Autodesk Inventor part; units mm, degrees
ref_plane "YZ Plane" through (0, 0, 0) normal (1, 0, 0) x (0, 1, 0)
ref_plane "XZ Plane" through (0, 0, 0) normal (0, 1, 0) x (-1, 0, 0)
ref_plane "XY Plane" through (0, 0, 0) normal (0, 0, 1) x (1, 0, 0)
sketch "Sketch12" plane through (0, 0, 0) normal (0, 0, 1) x (1, 0, 0)
  line L0 (-49, -21) -> (49, -21)
  line L1 (-49, 21) -> (-49, 9)
  line L2 (-49, -9) -> (-52, -9)
  line L3 (-52, -9) -> (-52, -3.75)
  line L4 (-52, 9) -> (-49, 9)
  line L5 (-49, -3.75) -> (-52, -3.75)
  line L6 (-49, 3.75) -> (-52, 3.75)
  line L7 (-44, -1.5) -> (-44, 1.5)
  line L8 (-49, 1.5) -> (-49, -1.5)
  line L9 (-49, -3.75) -> (-49, -9)
  line L10 (-49, 1.5) -> (-49, -1.5)
  line L11 (-49, 3.75) -> (-49, 1.5)
  line L12 (-47, -1.5) -> (-47, -2.65)
  line L13 (-44.6, -2.65) -> (-47, -2.65)
  line L14 (-44.6, -2.65) -> (-44.6, -1.5)
  line L15 (-44.6, 1.5) -> (-44.6, 2.65)
  line L16 (-47, 2.65) -> (-44.6, 2.65)
  line L17 (-47, 1.5) -> (-47, 2.65)
  line L18 (-49, -1.5) -> (-47, -1.5)
  line L19 (-44.6, -1.5) -> (-44, -1.5)
  line L20 (-44, 1.5) -> (-44.6, 1.5)
  line L21 (-47, 1.5) -> (-49, 1.5)
  line L22 (0, -30) -> (0, 33) construction
  line L23 (33.1667, 21) -> (33.1667, 24)
  line L24 (33.1667, 24) -> (5, 24)
  line L25 (-33.1667, 24) -> (-33.1667, 21)
  line L26 (-33.1667, 21) -> (-49, 21)
  line L27 (33.1667, 21) -> (49, 21)
  line L28 (-5, 21) -> (-5, 24)
  line L29 (5, 21) -> (5, 24)
  line L30 (-1.5, 21) -> (-1.5, 19)
  line L31 (-2.65, 19) -> (-1.5, 19)
  line L32 (-2.65, 19) -> (-2.65, 16.6)
  line L33 (-2.65, 16.6) -> (-1.5, 16.6)
  line L34 (-1.5, 16.6) -> (-1.5, 16)
  line L35 (-1.5, 16) -> (1.5, 16)
  line L36 (1.5, 16) -> (1.5, 16.6)
  line L37 (2.65, 16.6) -> (1.5, 16.6)
  line L38 (2.65, 16.6) -> (2.65, 19)
  line L39 (1.5, 19) -> (2.65, 19)
  line L40 (1.5, 19) -> (1.5, 21)
  line L41 (1.5, 21) -> (5, 21)
  line L42 (-5, 24) -> (-33.1667, 24)
  line L43 (5, 24) -> (-5, 24)
  line L44 (-1.5, 21) -> (-5, 21)
  circle A0 centre (0, 0) radius 11.5
  circle A1 centre (32, 0) radius 3.9
  circle A2 centre (-32, 0) radius 3.9
  line L45 (2.65, 19) -> (2.65, 16.6)
  line L46 (2.65, 16.6) -> (-2.65, 16.6)
  line L47 (-2.65, 16.6) -> (-2.65, 19)
  line L48 (-2.65, 19) -> (2.65, 19)
  line L49 (44.6, 2.65) -> (47, 2.65)
  line L50 (47, 2.65) -> (47, -2.65)
  line L51 (47, -2.65) -> (44.6, -2.65)
  line L52 (44.6, -2.65) -> (44.6, 2.65)
  line L53 (-44.6, 2.65) -> (-44.6, -2.65)
  line L54 (-44.6, -2.65) -> (-47, -2.65)
  line L55 (-47, -2.65) -> (-47, 2.65)
  line L56 (-47, 2.65) -> (-44.6, 2.65)
  circle A3 centre (-15.5, -15.5) radius 1.4
  circle A4 centre (-15.5, 15.5) radius 1.4
  circle A5 centre (15.5, 15.5) radius 1.4
  circle A6 centre (15.5, -15.5) radius 1.4
  line L57 (-52, -21) -> (52, -21)
  line L58 (52, -21) -> (52, -10.5)
  line L59 (52, -10.5) -> (49, -10.5)
  line L60 (49, -10.5) -> (49, 10.5)
  line L61 (49, 10.5) -> (52, 10.5)
  line L62 (52, 10.5) -> (52, 24)
  line L63 (52, 24) -> (34.6667, 24)
  line L64 (34.6667, 24) -> (34.6667, 21)
  line L65 (34.6667, 21) -> (-34.6667, 21)
  line L66 (-34.6667, 21) -> (-34.6667, 24)
  line L67 (-34.6667, 24) -> (-52, 24)
  line L68 (-52, 24) -> (-52, 10.5)
  line L69 (-52, 10.5) -> (-49, 10.5)
  line L70 (-49, 10.5) -> (-49, -10.5)
  line L71 (-49, -10.5) -> (-52, -10.5)
  line L72 (-52, -10.5) -> (-52, -21)
  line L73 (-52, -3.75) -> (-52, 3.75)
  line L74 (-52, 3.75) -> (-52, 9)
  line L75 (-72.8, 0) -> (72.8, 0) construction
  line L76 (-49, -9) -> (-49, -21)
  line L77 (-49, 9) -> (-49, 3.75)
  line L78 (-49, -1.5) -> (-49, -3.75)
  line L79 (49, 21) -> (49, 9)
  line L80 (49, -9) -> (52, -9)
  line L81 (52, -9) -> (52, -3.75)
  line L82 (52, 9) -> (49, 9)
  line L83 (49, -3.75) -> (52, -3.75)
  line L84 (49, 3.75) -> (52, 3.75)
  line L85 (44, -1.5) -> (44, 1.5)
  line L86 (49, -3.75) -> (49, -9)
  line L87 (49, 1.5) -> (49, -1.5)
  line L88 (49, 3.75) -> (49, 1.5)
  line L89 (47, -1.5) -> (47, -2.65)
  line L90 (44.6, -2.65) -> (47, -2.65)
  line L91 (44.6, -2.65) -> (44.6, -1.5)
  line L92 (44.6, 1.5) -> (44.6, 2.65)
  line L93 (47, 2.65) -> (44.6, 2.65)
  line L94 (47, 1.5) -> (47, 2.65)
  line L95 (49, -1.5) -> (47, -1.5)
  line L96 (44.6, -1.5) -> (44, -1.5)
  line L97 (44, 1.5) -> (44.6, 1.5)
  line L98 (47, 1.5) -> (49, 1.5)
  line L99 (52, -3.75) -> (52, 3.75)
  line L100 (52, 3.75) -> (52, 9)
  line L101 (49, -9) -> (49, -21)
  line L102 (49, 9) -> (49, 3.75)
  line L103 (49, -1.5) -> (49, -3.75)
  point P0 (0, 0)
  dimension "d102" = 3
  dimension "d103" = 5
  dimension "d108" = 3
  dimension "d109" = 5
  dimension "d113" = 1.5
  dimension "d114" = 1.5
  dimension "d115" = 10
  dimension "d116" = 5.3
  dimension "d117" = 7.5
extrude "Extrusion9" add sketch "Sketch12" along normal blind 3 contours L76 L70 L9 L18 L12 L13 L14 L19 L7 L20 L15 L16 L17 L21 L11 L1 L26 L65 L44 L30 L31 L32 L33 L34 L35 L36 L37 L38 L39 L40 L41 L27 L79 L60 L98 L50 L49 L52 L97 L85 L96 L51 L95 L101 L0 | L2 L3 L5 L9 | L60 L83 L81 L80 | L74 L4 L70 L6 | L84 L60 L82 L100 | L96 L85 L97 L52 | L25 L42 L28 L65 | L65 L29 L24 L23
properties part number "X-Motor-Housing_Front-Outer"
Check sheet for the modelled part. Datum: model origin and axes. Units: mm. A direction names the side the tool comes from. Coordinates: 2 decimals unless noted, no trailing zeros. Write each loop counter-clockwise with the first axis right and the second up, starting at its lowest first coordinate (ties: lowest second). Pieces come first, ordered by that corner, then holes. Notation, with made-up numbers: M -7,4.5 L 23,4.5 A16 ccw 23,28.5 Z; hole C 85,35 d11. An arc over 180 degrees is marked long. Answer as CSV lines item,"result".
Q1. Material ranges on probe 1 along Y at (x, z) = (15.5, 1.4); probe 2 along Y at (x, z) = (-45, 2.6); probe 3 along X at (y, z) = (3.5, 2.8), recorded low to high. Write a range as from..to.
Check result:
probe 1,"-21..-16.9, -14.1..14.1, 16.9..24"
probe 2,"-21..-2.65, 2.65..21"
probe 3,"-49..-33.72, -30.28..-10.95, 10.95..30.28, 33.72..49"
Q2. Cross-section at D-D (x = -32). Record the boundary of the cut face in (y, z), then the cut area to 3 significant figures.
Check result:
outline,"M -21,0 L -3.9,0 L -3.9,3 L -21,3 Z; M 3.9,0 L 24,0 L 24,3 L 3.9,3 Z"
area,"112 mm^2"
Q3. Go/stop test with flat-tipped pins: pin 1 (0.9 mm diameter, centred on x = -50, z = 1.5, fed in from -Y); pin 2 (1.3 mm diameter, centred on x = 2, z = 1, fed in from +Y); pin 3 (1 mm diameter, centred on y = 16.5, z = 1.5, fed in from +X); pin 4 (2 mm diameter, centred on x = -15.5, y = 15.5, fed in from +Z). Record where each tip stops, or that it passes through.
Check result:
pin 1,"y = -9"
pin 2,"y = 21"
pin 3,"x = 49"
pin 4,"through"
Q4. Set-up check for faces 4 (the face through (44.6, 0, 1)), 5 (the face through (-3, 21, 1)), 6 (the face through (41, 21, 1)), 7 (the face through (-49, 3, 1)), 8 (the face through (-49, -15, 1)): record each of +Z, -Z, +X, -X, +Y, -Y from which the full face is reachable in a straight line by a thin tool's end or side.
Check result:
face 4,"+Z, -Z"
face 5,"+Z, -Z, +Y"
face 6,"+Z, -Z, +X, +Y"
face 7,"+Z, -Z, -X"
face 8,"+Z, -Z, -X, -Y"
Q5. Mould release check, pull along Y, two halves, no side actions. Record for faces 1 (the face through (46, -2.65, 1)), 2 (the face through (5, 22, 1)), 3 (the face through (50, -9, 1)): released by +Y, released by -Y, zero draft, split by the parting line, or undercut.
Check result:
face 1,"undercut"
face 2,"zero draft"
face 3,"released by -Y"
Q6. Cross-section at A-A (y = 0). Record the boundary of the cut face in (x, z), then the cut area to 3 significant figures.
Check result:
outline,"M -44,0 L -35.9,0 L -35.9,3 L -44,3 Z; M -28.1,0 L -11.5,0 L -11.5,3 L -28.1,3 Z; M 11.5,0 L 28.1,0 L 28.1,3 L 11.5,3 Z; M 35.9,0 L 44.6,0 L 44.6,3 L 35.9,3 Z"
area,"150 mm^2"
Q7. Cross-section at B-B (x = 15.5). Record the boundary of the cut face in (y, z).
Check result:
outline,"M -21,0 L -16.9,0 L -16.9,3 L -21,3 Z; M -14.1,0 L 14.1,0 L 14.1,3 L -14.1,3 Z; M 16.9,0 L 24,0 L 24,3 L 16.9,3 Z"
Q8. Cross-section at C-C (y = 20). Record the boundary of the cut face in (x, z).
Check result:
outline,"M -49,0 L -1.5,0 L -1.5,3 L -49,3 Z; M 1.5,0 L 49,0 L 49,3 L 1.5,3 Z"
